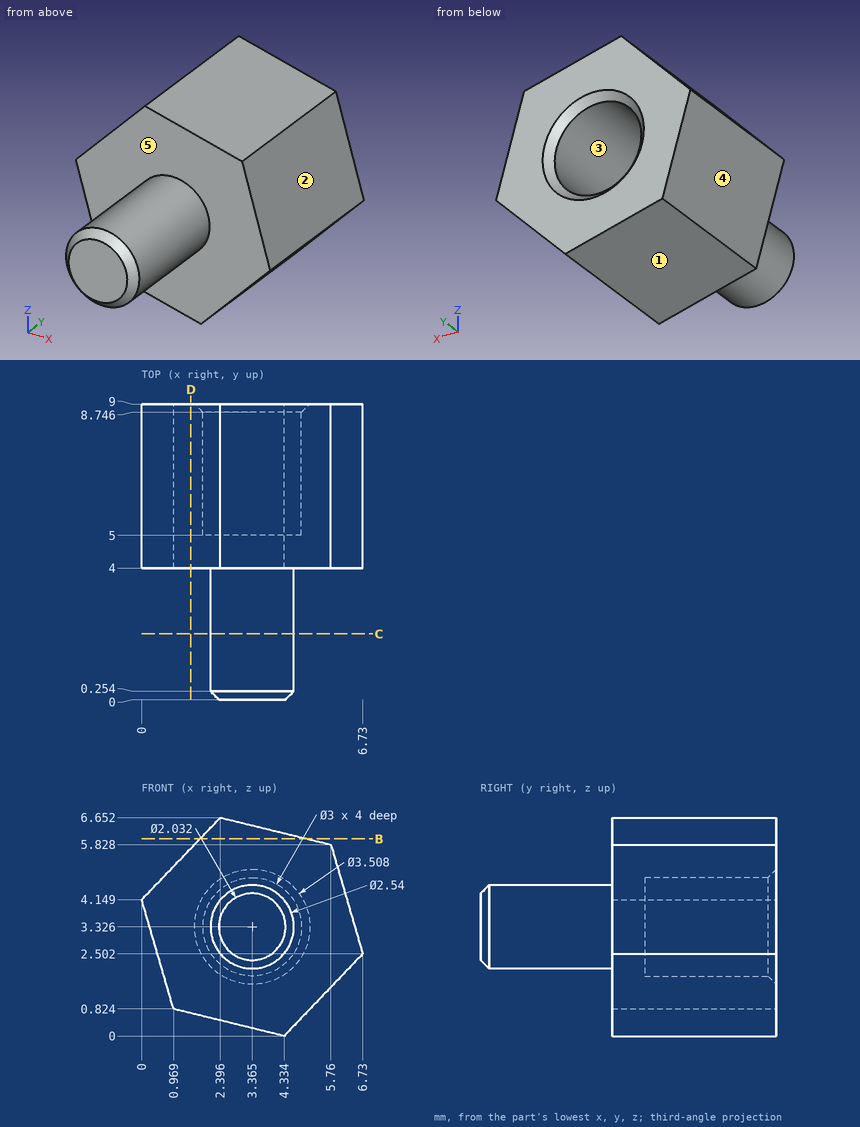
Here's the drawing with two shaded views (mm, measured from the low corner). I have some questions. A direction names the side the tool comes from. Round coordinates to 2 decimals unless told otherwise and drop trailing zeros. Loops run counter-clockwise (first coordinate to the right, second up) from the corner with the lowest first, then second, coordinate; pieces in that order, holes last. Notation, with made-up numbers: M 89,73.5 L 101,73.5 A16 cw 101,82.5 Z; hole C 19.25,-17.5 d8. An arc over 180 degrees is marked long. Answer as a JSON object with one key per item and string values. Group by question number.
Q1. On a 3-axis mill with a long thin cutter (end or side, diameter ignored), from which of +Z, -Z, +X, -X, +Y, -Y can I reach the whole of each face in a straight line? I mean the marked faces 4 and 5. Say none if no direction works.
Q2. Please list where these lines run through material, in increasing order: L1, parallel to X at y = 2.75, z = 3.25; L2, parallel to Z at x = 3.25, y = 8 (1 decimal); L3, parallel to Z at x = 4.5, y = 5.5 (1 decimal).
Q3. We'd pull the mould along X, two halves only. Please class the marked faces 1, 2 and 3: +X half, -X half, draft (parallel to the pull), parting line (faces both ways), or undercut.
Q4. Will these pins go through, and if not, where does the flat tip stop? pin 1 (0.9 mm diameter, centred on x = 3, z = 3, fed in from +Y); pin 2 (2 mm diameter, centred on y = 2.5, z = 1.5, fed in from +X); pin 3 (3 mm diameter, centred on x = 1, y = 7.5, fed in from +Z); pin 4 (4 mm diameter, centred on x = 1.5, y = 8, fed in from -Z).
Q5. Imagine slicing it at D-D, the plane x = 1.5. Please give me the cut outline in (y, z), then the cut area to 3 significant figures.
Q6. Imagine slicing it at B-B, the plane z = 6. Please give me the cut outline in (x, y).
Q7. Imagine slicing it at C-C, the plane y = 2. Please give me the cut outline in (x, z) (1 decimal).
Findings:
{
 "1": {"face 4": "-Z, -X, +Y, -Y", "face 5": "-Y"},
 "2": {"L1": "x = 2.1 to 4.63", "L2": "z = 0.3 to 1.8, 4.8 to 6.4", "L3": "z = 0.2 to 2.3, 4.3 to 6.1"},
 "3": {"face 1": "-X half", "face 2": "+X half", "face 3": "undercut"},
 "4": {"pin 1": "stops at y = 5", "pin 2": "stops at x = 4.33", "pin 3": "stops at z = 6.65", "pin 4": "stops at z = 0.2"},
 "5": {"outline": "M 4,0.69 L 9,0.69 L 9,5.72 L 4,5.72 Z", "area": "25.1 mm2"},
 "6": {"outline": "M 1.77,4 L 5.06,4 L 5.06,9 L 1.77,9 Z"},
 "7": {"outline": "C 3.4,3.3 d2.5"}
}
